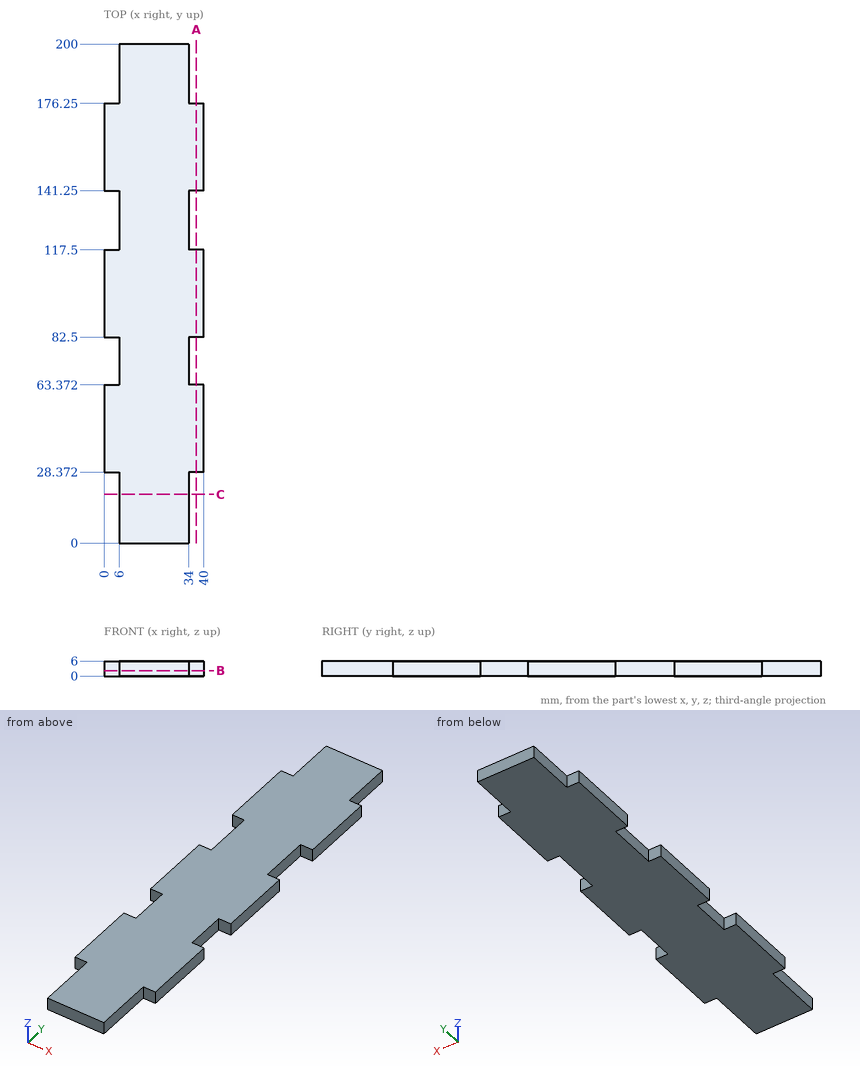
Study the drawing (mm; zero at the part's minimum x, y, z) and answer. Coordinates: 2 decimals unless noted, no trailing zeros. Write each loop counter-clockwise with the first axis right and the second up, starting at its lowest first coordinate (ties: lowest second). Pieces come first, ordered by that corner, then holes. Notation, with made-up numbers: (45.25, 24) - (89.25, 24) arc R13 cw to (89.25, 45) - close; hole circle Ø6 at (-29.75, 27.25). An arc over 180 degrees is marked (long way). Answer as a JSON object with one key per item and string values.
Q1. Find section A-A (x = 37). Write down the section's boundary in (y, z), plus the area to 3 significant figures.
Results list:
{"outline": "(28.37, 0) - (63.37, 0) - (63.37, 6) - (28.37, 6) - close; (82.5, 0) - (117.5, 0) - (117.5, 6) - (82.5, 6) - close; (141.25, 0) - (176.25, 0) - (176.25, 6) - (141.25, 6) - close", "area": "630 mm^2"}
Q2. Consider L1, parallel to Y at x = 2, z = 1.05; L2, parallel to X at y = 126, z = 3.25. Determine where each line is inside the solid, lowest interval first. Write a range as from..to.
Results list:
{"L1": "y = 28.37..63.37, 82.5..117.5, 141.25..176.25", "L2": "x = 6..34"}
Q3. Find section B-B (z = 2.2). Write down the section's boundary in (x, y).
Results list:
{"outline": "(0, 28.37) - (6, 28.37) - (6, 0) - (34, 0) - (34, 28.37) - (40, 28.37) - (40, 63.37) - (34, 63.37) - (34, 82.5) - (40, 82.5) - (40, 117.5) - (34, 117.5) - (34, 141.25) - (40, 141.25) - (40, 176.25) - (34, 176.25) - (34, 200) - (6, 200) - (6, 176.25) - (0, 176.25) - (0, 141.25) - (6, 141.25) - (6, 117.5) - (0, 117.5) - (0, 82.5) - (6, 82.5) - (6, 63.37) - (0, 63.37) - close"}
Q4. Find section C-C (y = 19.5). Write down the section's boundary in (x, z), plus the area to 3 significant figures.
Results list:
{"outline": "(6, 0) - (34, 0) - (34, 6) - (6, 6) - close", "area": "168 mm^2"}
Q5. Given pin 1 Ø1.8 at (x, z) = (2, 3.5) entering from -Y; pin 2 Ø3 at (x, z) = (2, 4) entering from +Y; pin 3 Ø1.8 at (y, z) = (185.5, 4.5) entering from -X; pin 4 Ø2 at (x, y) = (16.5, 171.5) entering from -Z, each flat-ended and moving along its own axis, determine where each tip first touches the part or whether it passes through.
Results list:
{"pin 1": "stops at y = 28.37", "pin 2": "stops at y = 176.25", "pin 3": "stops at x = 6", "pin 4": "stops at z = 0"}
